```python
from build123d import *

# Parameters (mm, degrees)
SKETCH1_R           = 6.35
BOSS_EXTRUDE1_DEPTH = 25.4
SKETCH2_R           = 3.96875
BOSS_EXTRUDE2_DEPTH = 50.8
FILLET1_R           = 6.35


with BuildPart() as part:
    # Sketch1 → Boss-Extrude1 (new, symmetric)
    with BuildSketch(Plane.XY):
        Circle(SKETCH1_R)
    extrude(amount=BOSS_EXTRUDE1_DEPTH, both=True)

    # Sketch2 → Boss-Extrude2 (add, symmetric)
    with BuildSketch(Plane.XY):
        Circle(SKETCH2_R)
    extrude(amount=BOSS_EXTRUDE2_DEPTH, both=True)

    # Fillet1
    # the kernel refuses this fillet: 6.35 mm, written as the material it adds along each edge
    with BuildSketch(Plane(origin=(0, 0, -25.4), x_dir=(1, 0, 0), z_dir=(0, -1, 0))) as fillet1_piece_1:
        with BuildLine():
            CenterArc((10.31875, -4.956967161), FILLET1_R, 128.682187453, 51.317812547)
            Line((3.96875, -4.956967161), (3.84175, -4.956967161))
            Line((3.84175, -4.956967161), (3.84175, 0))
            Line((3.84175, 0), (3.96875, 0.127))
            ThreePointArc((3.96875, 0.127), (5.159375, 0.127), (6.270625, 0.099139343))
            Line((6.270625, 0.099139343), (6.35, 0))
        make_face()
    revolve(axis=Axis((0, 0, -25.4), (0, 0, 1)))
    with BuildSketch(Plane(origin=(0, 0, 25.4), x_dir=(1, 0, 0), z_dir=(0, -1, 0))) as fillet1_piece_2:
        with BuildLine():
            CenterArc((10.31875, 4.956967161), FILLET1_R, 180, 51.317812547)
            Line((3.96875, 4.956967161), (3.84175, 4.956967161))
            Line((3.84175, 4.956967161), (3.84175, 0))
            Line((3.84175, 0), (3.96875, -0.127))
            ThreePointArc((3.96875, -0.127), (5.159375, -0.127), (6.270625, -0.099139343))
            Line((6.270625, -0.099139343), (6.35, 0))
        make_face()
    revolve(axis=Axis((0, 0, 25.4), (0, 0, 1)))


solid = part.part
```
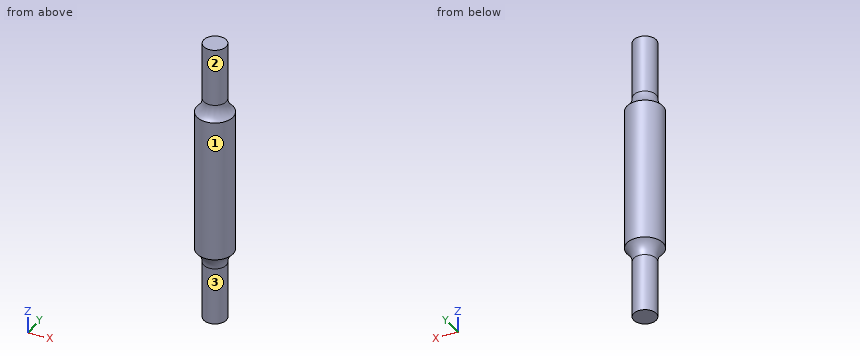
Verification items for the finished model (mm, model axes). Face numbers are marked on the shaded views. A direction names the side the tool comes from. Coordinates: 2 decimals unless noted, no trailing zeros. Loops run counter-clockwise (first coordinate to the right, second up) from the corner with the lowest first, then second, coordinate; pieces in that order, holes last. Notation, with made-up numbers: (38.5, 3) -> (72.5, 3) arc R26 ccw to (72.5, 31) -> close; hole circle Ø4 at (74.25, 60.25). An arc over 180 degrees is marked (long way). Answer in a Markdown table with one row per item. Add a question column.
1. Section check C-C, the plane z = -21. Enter the section's corners in (x, y).
2. Access from +Z, -Z, +X, -X, +Y, -Y to the whole of each face (thin tool, end or side, straight path). Record for the marked faces 1, 2 and 3.
3. Section check D-D, the plane z = 40.5. Enter the section's corners in (x, y).
4. Section check A-A, the plane y = 0. Enter the section's corners in (x, z), then the cut area to 3 significant figures.
5. Depth check by flat-ended pin: P1, Ø1, axis at x = -2, z = 39.5, coming from the +Y side. Enter the tip coordinate at first touch or a pass-through.
6. Material ranges on probe 1 along Y at (x, z) = (0, 38); probe 2 along Y at (x, z) = (0.25, -4.5); probe 3 along X at (y, z) = (1, 27), recorded low to high. Write a range as [from, to].
Derived:
| question | item | result |
|---|---|---|
| 1 | outline | circle Ø12.7 at (0, 0) |
| 2 | face 1 | +Z, -Z |
| 2 | face 2 | +Z |
| 2 | face 3 | -Z |
| 3 | outline | circle Ø7.94 at (0, 0) |
| 4 | outline | (-6.35, -25.4) arc R6.35 cw to (-3.97, -30.36) -> (-3.97, -50.8) -> (3.97, -50.8) -> (3.97, -30.36) arc R6.35 cw to (6.35, -25.4) -> (6.35, 25.4) arc R6.35 cw to (3.97, 30.36) -> (3.97, 50.8) -> (-3.97, 50.8) -> (-3.97, 30.36) arc R6.35 cw to (-6.35, 25.4) -> close |
| 4 | area | 1,060 mm² |
| 5 | P1 | stops at y = 3.67 |
| 6 | probe 1 | y = [-3.97, 3.97] |
| 6 | probe 2 | y = [-6.35, 6.35] |
| 6 | probe 3 | x = [-4.83, 4.83] |
